The model under review builds one solid part; all positions refer to its coordinate system, in mm. A direction names the side the tool comes from. Coordinates: 2 decimals unless noted, no trailing zeros. Loops run counter-clockwise (first coordinate to the right, second up) from the corner with the lowest first, then second, coordinate; pieces in that order, holes last. Notation, with made-up numbers: M 69.5,49 L 115.5,49 A19 cw 115.5,80 Z; hole C 48,56.5 d1. An arc over 180 degrees is marked long. Use one line per item in the form item = value.
```python
from build123d import *

# Parameters (mm, degrees)
F1_DEPTH = 50.8
F2_DEPTH = 25.4
F0_W     = 25.4
F0_H     = 25.4
F3_DEPTH = 25.4
F4_W     = 25.4
F4_H     = 25.4
F5_DEPTH = 101.6
F6_W     = 12.7
F6_H     = 12.7
F7_DEPTH = 38.1


with BuildPart() as f1:
    # F0 (on Top) → F1 (new body)
    with BuildSketch(Plane.XY):
        Polygon((-50.8, 55.880003), (-50.8, -55.880003), (-25.4, -55.880003), (25.4, -55.880003), (50.8, -55.880003), (50.8, 55.880003), (12.7, 55.880003), (-12.7, 55.880003), align=None)
    extrude(amount=F1_DEPTH)

    # F0 (on Top) → F2 (join)
    with BuildSketch(Plane.XY):
        Polygon((25.4, -55.880003), (-25.4, -55.880003), (-25.4, -68.580003), (-12.7, -68.580003), (12.7, -68.580003), (25.4, -68.580003), align=None)
    extrude(amount=F2_DEPTH)

    # F0 (on Top) → F3 (join)
    with BuildSketch(Plane.XY):
        with Locations((0, 68.580003)):
            Rectangle(F0_W, F0_H)
    extrude(amount=F3_DEPTH)

    # F4 (on face) → F5 (join)
    with BuildSketch(Plane.XZ.offset(55.880003)):
        with Locations((-63.5, 25.4)):
            Rectangle(F4_W, F4_H)
        with Locations((63.5, 25.4)):
            Rectangle(F4_W, F4_H)
    extrude(amount=-F5_DEPTH)

    # F6 (on face) → F7 (join)
    with BuildSketch(Plane(origin=(0, 0, 0), x_dir=(1, 0, 0), z_dir=(0, 0, -1))):
        with Locations((-44.45, -62.230003)):
            Rectangle(F6_W, F6_H)
        with Locations((44.45, -62.230003)):
            Rectangle(F6_W, F6_H)
    extrude(amount=-F7_DEPTH)


solid = f1.part
```
1. Add section C-C (y = -19.5). State the section outline as (x, z) points.
Response values:
outline = M -76.2,12.7 L -50.8,12.7 L -50.8,0 L 50.8,0 L 50.8,12.7 L 76.2,12.7 L 76.2,38.1 L 50.8,38.1 L 50.8,50.8 L -50.8,50.8 L -50.8,38.1 L -76.2,38.1 Z
2. Add section B-B (z = 30). State the section outline as (x, y) points.
Response values:
outline = M -76.2,-55.88 L 76.2,-55.88 L 76.2,45.72 L 50.8,45.72 L 50.8,68.58 L 38.1,68.58 L 38.1,55.88 L -38.1,55.88 L -38.1,68.58 L -50.8,68.58 L -50.8,45.72 L -76.2,45.72 Z
3. Insertion check: P1, Ø4, axis at y = 59.5, z = 28, coming from the +X side; P2, Ø12, axis at y = -27, z = 39.5, coming from the -X side; P3, Ø20.5, axis at x = -67, z = 19.5, coming from the +Y side; P4, Ø7.5, axis at x = 61, y = -15.5, coming from the +Z side. Each pin has a flat end and moves straight along its axis. Give the tip position at first contact, or say it passes through.
Response values:
P1 = 50.8
P2 = -76.2
P3 = 45.72
P4 = 38.1
4. Add section A-A (y = 64). State the section outline as (x, z) points, then the cut area to 3 significant figures.
Response values:
outline = M -50.8,0 L -38.1,0 L -38.1,38.1 L -50.8,38.1 Z; M -12.7,0 L 12.7,0 L 12.7,25.4 L -12.7,25.4 Z; M 38.1,0 L 50.8,0 L 50.8,38.1 L 38.1,38.1 Z
area = 1,610 mm^2
5. Machinability: for faces 4 (the face through (-45, 62, 38.1)), 5 (the face through (38.1, 62, 19)), 6 (the face through (-45, 68.58, 19)), which of the approach directions +Z, -Z, +X, -X, +Y, -Y give a long, thin tool a straight path to every point of the face, cutting with its end or side? Answer none if there is none.
Response values:
face_4 = +Z, +X, -X, +Y
face_5 = +Z, -Z, +Y
face_6 = +Z, -Z, -X, +Y
6. Add section D-D (x = -43.5). State the section outline as (y, z) points.
Response values:
outline = M -55.88,0 L 68.58,0 L 68.58,38.1 L 55.88,38.1 L 55.88,50.8 L -55.88,50.8 Z
7. The part is to be moulded in two halves that separate along X. For faces 1 (the face through (-38.1, 62, 19)), 2 (the face through (-76.2, -6, 25)), 3 (the face through (-64, 45.72, 26)), say which applies: pulls with the +X half, pulls with the -X half, needs draft (parallel to the pull), parting line crosses it, or undercut.
Response values:
face_1 = undercut
face_2 = pulls with the -X half
face_3 = needs draft
8. Wall thickness on line 1 along Y through (x, z) = (-5.5, 48); line 2 along X through (y, z) = (54, 9.5); line 3 along Y through (x, z) = (70.5, 31.5): over which ranges is each line inside the solid? List them lowest first. Write a range as from..to.
Response values:
line_1 = -55.88..55.88
line_2 = -50.8..50.8
line_3 = -55.88..45.72
